from build123d import *

# Parameters (mm, degrees)
F2_R = 2.5281634783
F5_R = 1.8773668217


with BuildPart() as f1:
    # F0 (on Front) → F1 (revolve)
    with BuildSketch(Plane.XZ):
        Polygon((-12.0703522116, 0), (-44.3681403995, 32.4136614799), (-44.3681403995, 0), align=None)
    revolve(axis=Axis((-44.3681403995, 0, 16.20683074), (0, 0, -1)))

    # F2
    f2_edges = [f1.edges().sort_by_distance(p)[0] for p in [
        (-76.665929, 0, 0),
        (-28.219246, 0, 16.206831),
    ]]
    fillet(f2_edges, radius=F2_R)

    # F3 (on Front) → F4 (revolve)
    with BuildSketch(Plane.XZ):
        Polygon((-44.6098931134, 62.4538473785), (-44.6098931134, 31.946439296), (-19.2829854786, 62.4538473785), align=None)
    revolve(axis=Axis((-44.6098931134, 0, 47.2001433372), (0, 0, 1)))

    # F5
    f5_edges = [f1.edges().sort_by_distance(p)[0] for p in [
        (-69.936801, 0, 62.453847),
    ]]
    fillet(f5_edges, radius=F5_R)


solid = f1.part
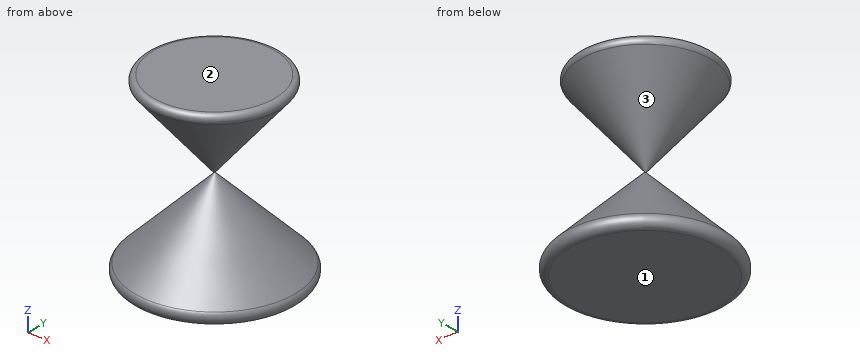
Input: part model. Units: mm. Frame: model coordinates. Face numbers are marked on the shaded views. Round coordinates to 2 decimals unless told otherwise and drop trailing zeros. Loops run counter-clockwise (first coordinate to the right, second up) from the corner with the lowest first, then second, coordinate; pieces in that order, holes last. Notation, with made-up numbers: (49.5, 52) -> (89.5, 52) arc R17 ccw to (89.5, 84) -> close; hole circle Ø9 at (31.25, 50). An arc over 180 degrees is marked (long way). Answer as a JSON object with one key per item and string values. Group by question number.
1) Section query B-B on z = 27. Output: boundary loops of the cut face in (x, y), plus the area to 3 significant figures.
2) Section query A-A on z = 51.5. Output: boundary loops of the cut face in (x, y).
3) Draft query along Z for the marked faces 1, 2 and 3. Return one class per face: +Z half, -Z half, draft (parallel to the pull), parting line (faces both ways), or undercut.
4) Pin query (flat end, axial travel): pin 1 (1 mm diameter, centred on x = -36.5, z = 7, fed in from -Y); pin 2 (1.5 mm diameter, centred on x = -37.5, z = 24.5, fed in from -Y); pin 3 (2 mm diameter, centred on y = 4.5, z = 30.5, fed in from -X); pin 4 (6 mm diameter, centred on y = 2.5, z = 41, fed in from -X). Return the tip coordinate at first contact, or that it passes through.
5) Ray query, L1, parallel to X at y = -5.5, z = 3.5; L2, parallel to Z at x = -49.5, y = 0; L3, parallel to Z at x = -61, y = -4.5. Return the intervals inside material, ascending.
Reply:
{
 "1": {"outline": "circle Ø10.79 at (-44.37, 0)", "area": "91.4 mm2"},
 "2": {"outline": "circle Ø32.47 at (-44.61, 0)"},
 "3": {"face 1": "-Z half", "face 2": "+Z half", "face 3": "undercut"},
 "4": {"pin 1": "stops at y = -24.62", "pin 2": "stops at y = -5.55", "pin 3": "passes through", "pin 4": "stops at x = -54.38"},
 "5": {"L1": "x = -72.38 to -16.36", "L2": "z = 0 to 27.26, 37.84 to 62.45", "L3": "z = 0 to 15.12, 52.42 to 62.45"}
}
